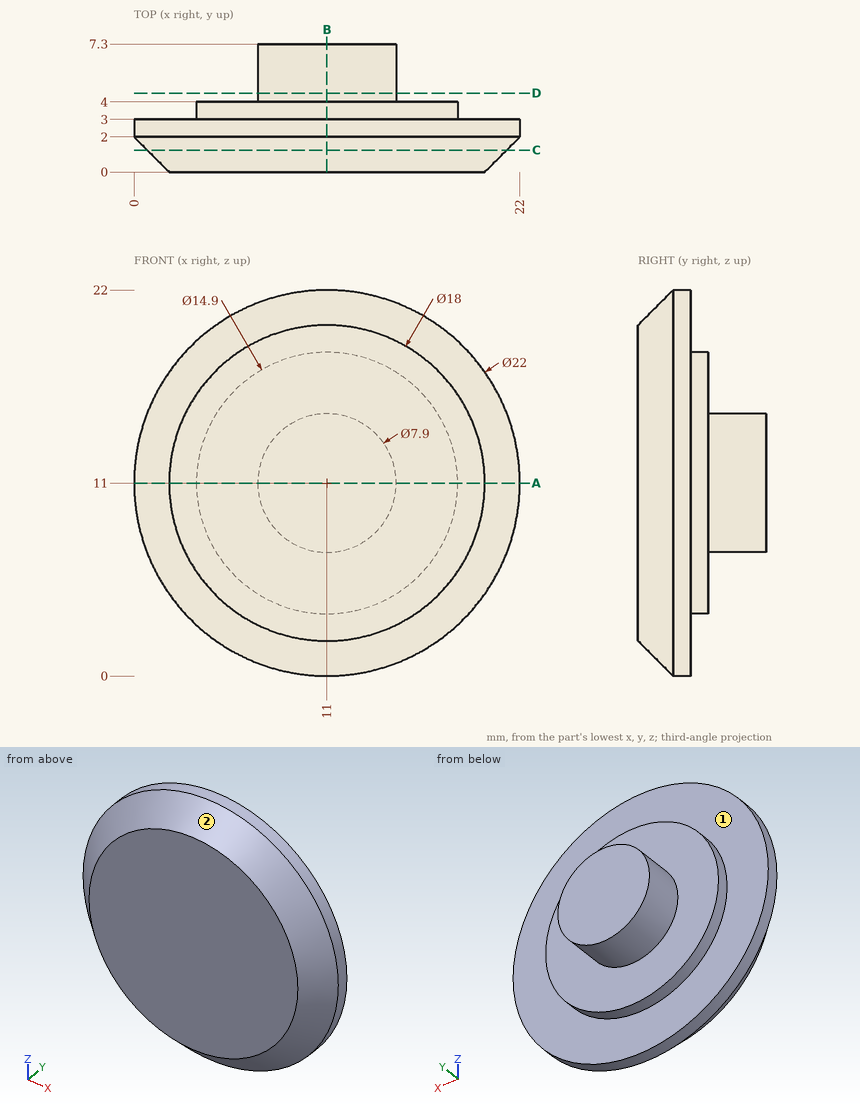
Input: dimensioned drawing with shaded views. Units: mm. Origin: part minimum x, y, z. A direction names the side the tool comes from. Give positions to 0.01 mm unless a question says otherwise; leave off trailing zeros. Order: outer loops, then holes, each group sorted by start corner. A loop starts at its lowest first (then second) coordinate and runs counter-clockwise, first axis right, second up. Notation, with made-up numbers: (81, -1.75) -> (106, -1.75) arc R21 ccw to (106, 24.25) -> close; hole circle Ø3 at (79.5, -21.75). An arc over 180 degrees is marked (long way). Use a Markdown table: item, result.
1) Section query D-D, the plane y = 4.5. Return the cut outline in (x, z).
Answer list:
| item | result |
|---|---|
| outline | circle Ø7.9 at (11, 11) |
2) Contact query for flat-ended pins moving along their axis: P1, Ø5, axis at x = 10, z = 4, coming from the +Y side; P2, Ø2, axis at x = 5.5, z = 4.5, coming from the +Y side; P3, Ø1.5, axis at y = 3, z = 7, coming from the -X side; P4, Ø2, axis at x = 6, y = 6.5, coming from the +Z side (3 decimals). Output: stop coordinate, or through.
Answer list:
| item | result |
|---|---|
| P1 | y = 4 |
| P2 | y = 3 |
| P3 | x = 0.49 |
| P4 | through |
3) Section query A-A, the plane z = 11. Return the cut outline in (x, y), then the cut area to 3 significant figures.
Answer list:
| item | result |
|---|---|
| outline | (0, 2) -> (2, 0) -> (20, 0) -> (22, 2) -> (22, 3) -> (18.45, 3) -> (18.45, 4) -> (14.95, 4) -> (14.95, 7.3) -> (7.05, 7.3) -> (7.05, 4) -> (3.55, 4) -> (3.55, 3) -> (0, 3) -> close |
| area | 103 mm² |
4) Section query B-B, the plane x = 11. Return the cut outline in (y, z).
Answer list:
| item | result |
|---|---|
| outline | (0, 2) -> (2, 0) -> (3, 0) -> (3, 3.55) -> (4, 3.55) -> (4, 7.05) -> (7.3, 7.05) -> (7.3, 14.95) -> (4, 14.95) -> (4, 18.45) -> (3, 18.45) -> (3, 22) -> (2, 22) -> (0, 20) -> close |
5) Reachability of the marked faces 1 and 2 from +Z, -Z, +X, -X, +Y, -Y: full face, straight path, thin tool, end or side. Return the list, or none.
Answer list:
| item | result |
|---|---|
| face 1 | +Y |
| face 2 | -Y |
6) Section query C-C, the plane y = 1.25. Return the cut outline in (x, z), then the cut area to 3 significant figures.
Answer list:
| item | result |
|---|---|
| outline | circle Ø20.5 at (11, 11) |
| area | 330 mm² |
7) Ray query, line 1 along Y through (x, z) = (10, 18.5); line 2 along Y through (x, z) = (8.25, 5.5); line 3 along Z through (x, y) = (11, 3.5). Return the intervals inside material, ascending. Write a range as [from, to].
Answer list:
| item | result |
|---|---|
| line 1 | [0, 3] |
| line 2 | [0, 4] |
| line 3 | [3.55, 18.45] |
